Build history of the part. All positions in model axes, mm. A direction names the side the tool comes from. Round coordinates to 2 decimals unless told otherwise and drop trailing zeros. Loops run counter-clockwise (first coordinate to the right, second up) from the corner with the lowest first, then second, coordinate; pieces in that order, holes last. Notation, with made-up numbers: M 30,5 L 35,5 A29 ccw 35,34 Z; hole C 82,60 d3. An arc over 180 degrees is marked long. One line per item, written item: value.
```python
from build123d import *

# Parameters (mm, degrees)
SKETCH1_R           = 16
SKETCH1_R_2         = 8
BOSS_EXTRUDE1_DEPTH = 15
SKETCH2_R           = 16
BOSS_EXTRUDE2_DEPTH = 73
SKETCH2_3_R         = 8
BOSS_EXTRUDE3_DEPTH = 25
BOSS_EXTRUDE7_DEPTH = 73
CUT_EXTRUDE1_DEPTH  = 73


with BuildPart() as part:
    # Sketch1 → Boss-Extrude1 (new body)
    with BuildSketch(Plane(origin=(0, 0, 0), x_dir=(0, 1, 0), z_dir=(0, 0, 1))):
        with BuildLine():
            Line((-31.836853451, -3.227191092), (-20, -120))
            ThreePointArc((-20, -120), (0, -140), (20, -120))
            Line((20, -120), (31.836853451, -3.227191092))
            ThreePointArc((31.836853451, -3.227191092), (0, 32), (-31.836853451, -3.227191092))
        make_face()
        with Locations(Location((0, 0, 0), (0, 0, 270))):
            Circle(SKETCH1_R, mode=Mode.SUBTRACT)
        with Locations(Location((0, -120, 0), (0, 0, 270))):
            Circle(SKETCH1_R_2, mode=Mode.SUBTRACT)
    extrude(amount=BOSS_EXTRUDE1_DEPTH)

    # Sketch2 → Boss-Extrude2 (add)
    with BuildSketch(Plane.XY.offset(15)):
        with BuildLine():
            ThreePointArc((4.090932126, -31.749299027), (24.038632569, -21.139958812), (32.01177462, 0))
            ThreePointArc((32.01177462, 0), (24.038632569, 21.139958812), (4.090932126, 31.749299027))
            Line((4.090932126, 31.749299027), (3.227191092, 31.836853451))
            ThreePointArc((3.227191092, 31.836853451), (-32, 0), (3.227191092, -31.836853451))
            Line((3.227191092, -31.836853451), (4.090932126, -31.749299027))
        make_face()
        Circle(SKETCH2_R, mode=Mode.SUBTRACT)
    extrude(amount=BOSS_EXTRUDE2_DEPTH)

    # Sketch2<3> → Boss-Extrude3 (add)
    with BuildSketch(Plane.XY.offset(15)):
        with BuildLine():
            ThreePointArc((120, -20), (134.142135624, -14.142135624), (140, 0))
            ThreePointArc((140, 0), (134.142135624, 14.142135624), (120, 20))
            ThreePointArc((120, 20), (100, 0), (120, -20))
        make_face()
        with Locations((120, 0)):
            Circle(SKETCH2_3_R, mode=Mode.SUBTRACT)
    extrude(amount=BOSS_EXTRUDE3_DEPTH)

    # Sketch5 → Boss-Extrude7 (add)
    with BuildSketch(Plane.XY.offset(15)):
        with BuildLine():
            ThreePointArc((30.996027396, 8), (31.756822554, 4.032113045), (32.01177462, 0))
            Line((32.01177462, 0), (100, 0))
            ThreePointArc((100, 0), (100.421873741, 4.086192874), (101.66969722, 8))
            Line((101.66969722, 8), (30.996027396, 8))
        make_face()
        with BuildLine():
            Line((100, 0), (32.01177462, 0))
            ThreePointArc((32.01177462, 0), (31.756822554, -4.032113045), (30.996027396, -8))
            Line((30.996027396, -8), (101.66969722, -8))
            ThreePointArc((101.66969722, -8), (100.421873741, -4.086192874), (100, 0))
        make_face()
    extrude(amount=BOSS_EXTRUDE7_DEPTH)

    # Sketch6 → Cut-Extrude1 (cut)
    with BuildSketch(Plane.XZ.offset(8)):
        Polygon((30.996027396, 88), (101.66969722, 40), (101.66969722, 88), align=None)
    extrude(amount=-CUT_EXTRUDE1_DEPTH, mode=Mode.SUBTRACT)


solid = part.part
```
Item 1: Drop flat-ended pins along their axis: P1, Ø12, axis at y = -17.5, z = 34, coming from the +X side; P2, Ø3, axis at y = 7, z = 40.5, coming from the -X side; P3, Ø12, axis at x = 47, z = 18.5, coming from the -Y side. Give the stop position or say it passes through.
Check values:
P1: stops at x = 136.36
P2: stops at x = -31.52
P3: stops at y = -27.89
Item 2: Slice it at B-B, the plane z = 30. Give the cut face in (x, y).
Check values:
outline: M 3.23,-31.84 L 4.09,-31.75 A32.01 ccw 31,-8 L 101.67,-8 A20 ccw long 101.67,8 L 31,8 A32.01 ccw 4.09,31.75 L 3.23,31.84 A32 ccw long Z; hole C 0,0 d32; hole C 120,0 d16
Item 3: Slice it at A-A, the plane x = -8. Give the cut face in (y, z), and give its area (3 significant figures).
Check values:
outline: M -30.98,0 L -13.86,0 L -13.86,88 L -30.98,88 Z; M 13.86,0 L 30.98,0 L 30.98,88 L 13.86,88 Z
area: 3,010 mm2
Item 4: Slice it at D-D, the plane y = -6. Give the cut face in (x, z).
Check values:
outline: M -31.43,0 L -14.83,0 L -14.83,88 L -31.43,88 Z; M 14.83,0 L 114.71,0 L 114.71,40 L 100.92,40 L 100.92,40.51 L 31,88 L 14.83,88 Z; M 125.29,0 L 139.08,0 L 139.08,40 L 125.29,40 Z
Item 5: Wall check: line 1 along Y through (x, z) = (120, 29); line 2 along Y through (x, z) = (0, 63); line 3 along X through (y, z) = (5.5, 21). Give the ranges that are in metal, low to high.
Check values:
line 1: y = -20 to -8, 8 to 20
line 2: y = -32 to -16, 16 to 32
line 3: x = -31.52 to -15.02, 15.02 to 114.19, 125.81 to 139.23
Item 6: Which spindle directions (+Z, -Z, +X, -X, +Y, -Y) get a long thin tool onto all of the face, cutting with end or side? Do faces 1 (the face through (-3.47, -15.62, 43.38)), 2 (the face through (58, -8, 43)), 3 (the face through (61, 17, 15)). Say none if no direction does.
Check values:
face 1: +Z, -Z
face 2: +Z, -Y
face 3: +Z, +Y
Item 7: Slice it at C-C, the plane y = 13.5. Give the cut face in (x, z), and give its area (3 significant figures).
Check values:
outline: M -29.01,0 L -8.59,0 L -8.59,88 L -29.01,88 Z; M 8.59,0 L 134.76,0 L 134.76,40 L 105.24,40 L 105.24,15 L 29.03,15 L 29.03,88 L 8.59,88 Z
area: 5,920 mm2
Item 8: Pull direction Y, two halves, no side cores. Call faces 4 (the face through (53, 0, 0)), 5 (the face through (20.98, -24.18, 50.99)), 6 (the face through (127.63, 2.4, 19.72)): pulls with the +Y half, pulls with the -Y half, needs draft (parallel to the pull), parting line crosses it, or undercut.
Check values:
face 4: needs draft
face 5: pulls with the -Y half
face 6: undercut
